```python
from build123d import *

# Parameters (mm, degrees)
SKETCH1_W           = 65
SKETCH1_H           = 100
SKETCH1_R           = 4
SKETCH1_R_2         = 1.7
BOSS_EXTRUDE1_DEPTH = 24
SKETCH3_R           = 3.5
CUT_EXTRUDE1_DEPTH  = 22


with BuildPart() as part:
    # Sketch1 → Boss-Extrude1 (new body)
    with BuildSketch(Plane(origin=(0, 0, 0), x_dir=(1, 0, 0), z_dir=(0, 1, 0))):
        Rectangle(SKETCH1_W, SKETCH1_H)
        with Locations((-25.4, -40)):
            Circle(SKETCH1_R, mode=Mode.SUBTRACT)
        with Locations((25.4, -40)):
            Circle(SKETCH1_R, mode=Mode.SUBTRACT)
        with Locations((25.4, -14.6)):
            Circle(SKETCH1_R, mode=Mode.SUBTRACT)
        with Locations((-25.4, -14.6)):
            Circle(SKETCH1_R, mode=Mode.SUBTRACT)
        with Locations((-17.5, 5.4)):
            Circle(SKETCH1_R_2, mode=Mode.SUBTRACT)
        with Locations((17.5, 37.4)):
            Circle(SKETCH1_R_2, mode=Mode.SUBTRACT)
        with Locations((-17.5, 37.4)):
            Circle(SKETCH1_R_2, mode=Mode.SUBTRACT)
        with Locations((17.5, 5.4)):
            Circle(SKETCH1_R_2, mode=Mode.SUBTRACT)
        with Locations((25.4, 10.8)):
            Circle(SKETCH1_R, mode=Mode.SUBTRACT)
        with Locations((-25.4, 10.8)):
            Circle(SKETCH1_R, mode=Mode.SUBTRACT)
    extrude(amount=BOSS_EXTRUDE1_DEPTH)

    # Sketch3 → Cut-Extrude1 (cut)
    with BuildSketch(Plane.XZ):
        with Locations((-17.5, -5.4)):
            Circle(SKETCH3_R)
        with Locations((17.5, -5.4)):
            Circle(SKETCH3_R)
        with Locations((-17.5, -37.4)):
            Circle(SKETCH3_R)
        with Locations((17.5, -37.4)):
            Circle(SKETCH3_R)
    extrude(amount=-CUT_EXTRUDE1_DEPTH, mode=Mode.SUBTRACT)


solid = part.part
```
Model file for the job. Use its own axes, mm. A direction names the side the tool comes from. Round coordinates to 2 decimals unless told otherwise and drop trailing zeros. Write each loop counter-clockwise with the first axis right and the second up, starting at its lowest first coordinate (ties: lowest second). Pieces come first, ordered by that corner, then holes. Notation, with made-up numbers: (6.5, 14.5) -> (26.5, 14.5) arc R20 cw to (26.5, 32.5) -> close; hole circle Ø6 at (43, 39.25). An arc over 180 degrees is marked (long way). Answer as CSV lines item,"result".
1. Mould opens along X. For faces 1 (the face through (-32.5, 12, 1)), 2 (the face through (0, 12, -50)), 3 (the face through (17.04, 10.85, -33.93)) say: +X half, -X half, draft (parallel to the pull), parting line (faces both ways), or undercut.
Resolved:
face 1,"-X half"
face 2,"draft"
face 3,"undercut"
2. Slice it at B-B, the plane y = 15.25. State how many separate pieces and enclosed holes the cut face has, plus the area to 3 significant figures.
Resolved:
separate pieces,"1"
enclosed holes,"10"
area,"6,040 mm²"
3. Slice it at A-A, the plane z = 14.6. List the corners of the cut face in (x, y).
Resolved:
outline,"(-32.5, 0) -> (-29.4, 0) -> (-29.4, 24) -> (-32.5, 24) -> close; (-21.4, 0) -> (21.4, 0) -> (21.4, 24) -> (-21.4, 24) -> close; (29.4, 0) -> (32.5, 0) -> (32.5, 24) -> (29.4, 24) -> close"
4. Tool access for faces 4 (the face through (-17.96, 10.85, -33.93)), 5 (the face through (24.879, 11.832, 36.034)): list every direction of +Z, -Z, +X, -X, +Y, -Y with a clear straight run to the whole face (end or side of a thin tool).
Resolved:
face 4,"-Y"
face 5,"+Y, -Y"
5. Slice it at C-C, the plane x = 25.4. List the corners of the cut face in (y, z), plus the area to 3 significant figures.
Resolved:
outline,"(0, -50) -> (24, -50) -> (24, -14.8) -> (0, -14.8) -> close; (0, -6.8) -> (24, -6.8) -> (24, 10.6) -> (0, 10.6) -> close; (0, 18.6) -> (24, 18.6) -> (24, 36) -> (0, 36) -> close; (0, 44) -> (24, 44) -> (24, 50) -> (0, 50) -> close"
area,"1,820 mm²"
6. Pin check, flat tip, straight feed: pin 1 Ø4.5 at (x, z) = (17.5, -5.4) entering from -Y. Stop position of the tip, or through.
Resolved:
pin 1,"y = 22"
7. Drill centre lines: line 1 (Z direction, x = 17.5, y = 22.55); line 2 (Z direction, x = 25.4, y = 7.5); line 3 (X direction, y = 11.25, z = 40). Where is each one in solid material? Low to high.
Resolved:
line 1,"-50 to -39.1, -35.7 to -7.1, -3.7 to 50"
line 2,"-50 to -14.8, -6.8 to 10.6, 18.6 to 36, 44 to 50"
line 3,"-32.5 to -29.4, -21.4 to 21.4, 29.4 to 32.5"
8. Slice it at D-D, the plane x = -17.5. List the corners of the cut face in (y, z), plus the area to 3 significant figures.
Resolved:
outline,"(0, -50) -> (24, -50) -> (24, -39.1) -> (22, -39.1) -> (22, -40.9) -> (0, -40.9) -> close; (0, -33.9) -> (22, -33.9) -> (22, -35.7) -> (24, -35.7) -> (24, -7.1) -> (22, -7.1) -> (22, -8.9) -> (0, -8.9) -> close; (0, -1.9) -> (22, -1.9) -> (22, -3.7) -> (24, -3.7) -> (24, 50) -> (0, 50) -> close"
area,"2,080 mm²"
